from build123d import *

# Parameters (mm, degrees)
SKETCH1_R           = 27
SKETCH1_R_2         = 17.5
BOSS_EXTRUDE1_DEPTH = 3
SKETCH2_R           = 2.05
CUT_EXTRUDE1_DEPTH  = 39.301436004
CIRPATTERN1_COUNT   = 8


with BuildPart() as part:
    # Sketch1 → Boss-Extrude1 (new body)
    with BuildSketch(Plane(origin=(0, 0, 0), x_dir=(1, 0, 0), z_dir=(0, 1, 0))):
        with Locations(Location((0, 0, 0), (0, 0, 270))):
            Circle(SKETCH1_R)
        with Locations(Location((0, 0, 0), (0, 0, 270))):
            Circle(SKETCH1_R_2, mode=Mode.SUBTRACT)
    extrude(amount=BOSS_EXTRUDE1_DEPTH)

    # Sketch2 → Cut-Extrude1 (cut, through all)
    with BuildSketch(Plane(origin=(0, 3, 0), x_dir=(1, 0, 0), z_dir=(0, 1, 0))):
        with Locations(Location((23, 0, 0), (0, 0, 270))):
            Circle(SKETCH2_R)
    cut_extrude1 = extrude(amount=-CUT_EXTRUDE1_DEPTH, mode=Mode.SUBTRACT)

    # CirPattern1: Cut-Extrude1 ×8 about axis
    cirpattern1_axis = Axis((0, 0, 0), (0, 1, 0))
    for i in range(1, CIRPATTERN1_COUNT):
        add(cut_extrude1.rotate(cirpattern1_axis, i * 360 / CIRPATTERN1_COUNT), mode=Mode.SUBTRACT)


solid = part.part
CAD build for the part. Positions are in the model's coordinates, mm. Coordinates: 2 decimals unless noted, no trailing zeros. Order: outer loops, then holes, each group sorted by start corner. A loop starts at its lowest first (then second) coordinate and runs counter-clockwise, first axis right, second up.
Item 1: Drill centre lines: L1, parallel to X at y = 0.8, z = 0; L2, parallel to X at y = 1.6, z = 1; L3, parallel to X at y = 1.4, z = -5. Where is each one in solid material? Low to high.
Check sheet entries:
L1: x = -27 to -25.05, -20.95 to -17.5, 17.5 to 20.95, 25.05 to 27
L2: x = -26.98 to -24.79, -21.21 to -17.47, 17.47 to 21.21, 24.79 to 26.98
L3: x = -26.53 to -16.77, 16.77 to 26.53
Item 2: Band-saw the part on A-A on x = 0. List the corners of the cut face in (y, z).
Check sheet entries:
outline: (0, -27) - (3, -27) - (3, -25.05) - (0, -25.05) - close; (0, -20.95) - (3, -20.95) - (3, -17.5) - (0, -17.5) - close; (0, 17.5) - (3, 17.5) - (3, 20.95) - (0, 20.95) - close; (0, 25.05) - (3, 25.05) - (3, 27) - (0, 27) - close
Item 3: Band-saw the part on C-C on y = 0.45. Give the number of separate pieces and of enclosed holes in the cut face, plus the area to 3 significant figures.
Check sheet entries:
separate pieces: 1
enclosed holes: 9
area: 1,220 mm2
Item 4: Band-saw the part on B-B on z = 0. List the corners of the cut face in (x, y).
Check sheet entries:
outline: (-27, 0) - (-25.05, 0) - (-25.05, 3) - (-27, 3) - close; (-20.95, 0) - (-17.5, 0) - (-17.5, 3) - (-20.95, 3) - close; (17.5, 0) - (20.95, 0) - (20.95, 3) - (17.5, 3) - close; (25.05, 0) - (27, 0) - (27, 3) - (25.05, 3) - close
Item 5: Pin check, flat tips, straight feed: pin 1 Ø3.5 at (x, z) = (-23, 0) entering from -Y; pin 2 Ø1 at (y, z) = (2, -6) entering from +X. Stop position of each tip, or through.
Check sheet entries:
pin 1: passes through
pin 2: stops at x = 26.43
Item 6: Two-plate mould, pull along X, no slides. Class faces 1 (the face through (-24.4, 1.5, 1.5)), 2 (the face through (-18, 3, 0)), 3 (the face through (-26.36, 1.48, -5.85)): +X half, -X half, draft (parallel to the pull), parting line (faces both ways), or undercut.
Check sheet entries:
face 1: undercut
face 2: draft
face 3: parting line
Item 7: Band-saw the part on D-D on x = -23. List the corners of the cut face in (y, z), plus the area to 3 significant figures.
Check sheet entries:
outline: (0, -14.14) - (3, -14.14) - (3, -2.05) - (0, -2.05) - close; (0, 2.05) - (3, 2.05) - (3, 14.14) - (0, 14.14) - close
area: 72.6 mm2
